from build123d import *

# Parameters (mm, degrees)
SKETCH1_W           = 230
SKETCH1_H           = 30
BOSS_EXTRUDE1_DEPTH = 50
CUT_EXTRUDE1_DEPTH  = 50
SKETCH3_W           = 21.468304511
SKETCH3_H           = 50
CUT_EXTRUDE2_DEPTH  = 50
CUT_EXTRUDE3_DEPTH  = 50
SKETCH5_R           = 2
CUT_EXTRUDE4_DEPTH  = 50
SKETCH6_R           = 2
CUT_EXTRUDE5_DEPTH  = 50


with BuildPart() as part:
    # Sketch1 → Boss-Extrude1 (new body)
    with BuildSketch(Plane.XY):
        Rectangle(SKETCH1_W, SKETCH1_H)
    extrude(amount=BOSS_EXTRUDE1_DEPTH)

    # Sketch2 → Cut-Extrude1 (cut)
    with BuildSketch(Plane.XZ.offset(15)):
        Polygon((-115, 9.270509831), (-86.468304511, 0), (-115, 0), align=None)
    extrude(amount=-CUT_EXTRUDE1_DEPTH, mode=Mode.SUBTRACT)

    # Sketch3 → Cut-Extrude2 (cut)
    with BuildSketch(Plane.XZ.offset(15)):
        with Locations((104.265847745, 25)):
            Rectangle(SKETCH3_W, SKETCH3_H)
    extrude(amount=-CUT_EXTRUDE2_DEPTH, mode=Mode.SUBTRACT)

    # Sketch4 → Cut-Extrude3 (cut)
    with BuildSketch(Plane.XZ.offset(15)):
        Polygon((-115, 16.630745401), (-85.359613429, 7), (93.531695489, 7), (93.531695489, 50), (-115, 50), align=None)
    extrude(amount=-CUT_EXTRUDE3_DEPTH, mode=Mode.SUBTRACT)

    # Sketch5 → Cut-Extrude4 (cut)
    with BuildSketch(Plane(origin=(-8.256988343, 0, -25.412397091), x_dir=(-0.9510565162951533, 0, 0.3090169943749483), z_dir=(-0.3090169943749483, 0, -0.9510565162951534))):
        with Locations((97.236244458, 7.5)):
            Circle(SKETCH5_R)
        with Locations((97.236244458, -7.5)):
            Circle(SKETCH5_R)
    extrude(amount=-CUT_EXTRUDE4_DEPTH, mode=Mode.SUBTRACT)

    # Sketch6 → Cut-Extrude5 (cut)
    with BuildSketch(Plane(origin=(0, 0, 0), x_dir=(-1, 0, 0), z_dir=(0, 0, -1))):
        with Locations((-51.531695489, 0)):
            Circle(SKETCH6_R)
        with Locations((-59.531695489, 0)):
            Circle(SKETCH6_R)
        with Locations((-67.531695489, 0)):
            Circle(SKETCH6_R)
        with Locations((-75.531695489, 0)):
            Circle(SKETCH6_R)
        with Locations((-43.531695489, 0)):
            Circle(SKETCH6_R)
        with Locations((-35.531695489, 0)):
            Circle(SKETCH6_R)
        with Locations((-27.531695489, 0)):
            Circle(SKETCH6_R)
        with Locations((-19.531695489, 0)):
            Circle(SKETCH6_R)
        with Locations((-11.531695489, 0)):
            Circle(SKETCH6_R)
        with Locations((-3.531695489, 0)):
            Circle(SKETCH6_R)
        with Locations((4.468304511, 0)):
            Circle(SKETCH6_R)
        with Locations((12.468304511, 0)):
            Circle(SKETCH6_R)
    extrude(amount=-CUT_EXTRUDE5_DEPTH, mode=Mode.SUBTRACT)


solid = part.part
Verification items for the finished model (mm, model axes). Round coordinates to 2 decimals unless told otherwise and drop trailing zeros. Loops run counter-clockwise (first coordinate to the right, second up) from the corner with the lowest first, then second, coordinate; pieces in that order, holes last. Notation, with made-up numbers: (61.5, 29) - (113.5, 29) arc R20 ccw to (113.5, 36) - close; hole circle Ø10 at (83, 55.5). An arc over 180 degrees is marked (long way). Answer in a Markdown table with one row per item. Add a question column.
Q1. Material ranges on line 1 (Z direction, x = -22.5, y = -13); line 2 (Y direction, x = 51, z = 1), recorded low to high.
Q2. Release check for a two-part mould opening along X. For faces 1 (the face through (-12, 15, 5)), 2 (the face through (69.53, 0.09, 3.45)), 3 (the face through (-98.3, 8.9, 7.5)), 4 (the face through (-100.387, -0.21, 11.883)) record: pulls with the +X half, pulls with the -X half, needs draft (parallel to the pull), parting line crosses it, or undercut.
Q3. Section check C-C on z = 14.5. Enter the section's corners in (x, y), plus the area to 3 significant figures.
Q4. Gauge pin test, flat ends, axial feed: pin 1 (3 mm diameter, centred on x = 11.53, y = 0, fed in from -Z); pin 2 (1.5 mm diameter, centred on x = 31, z = 7.5, fed in from +Y); pin 3 (6.5 mm diameter, centred on x = 3.53, y = 0, fed in from +Z); pin 4 (5 mm diameter, centred on x = -86, y = 5, fed in from +Z). Record the tip position at first contact, or that the pin passes through.
Q5. Section check A-A on x = -72. Enter the section's corners in (y, z), plus the area to 3 significant figures.
Q6. Section check B-B on y = 0. State how many separate pieces and enclosed holes the cut face has, plus the area to 3 significant figures.
Found:
| question | item | result |
|---|---|---|
| 1 | line 1 | z = 0 to 7 |
| 1 | line 2 | y = -15 to -1.93, 1.93 to 15 |
| 2 | face 1 | needs draft |
| 2 | face 2 | undercut |
| 2 | face 3 | undercut |
| 2 | face 4 | pulls with the +X half |
| 3 | outline | (-115, -15) - (-108.44, -15) - (-108.44, 15) - (-115, 15) - close |
| 3 | area | 197 mm² |
| 4 | pin 1 | passes through |
| 4 | pin 2 | stops at y = 15 |
| 4 | pin 3 | stops at z = 7 |
| 4 | pin 4 | stops at z = 8.02 |
| 5 | outline | (-15, 0) - (15, 0) - (15, 7) - (-15, 7) - close |
| 5 | area | 210 mm² |
| 6 | separate pieces | 13 |
| 6 | enclosed holes | 0 |
| 6 | area | 1,130 mm² |
